Model file for the job. Use its own axes, mm. A direction names the side the tool comes from. Round coordinates to 2 decimals unless told otherwise and drop trailing zeros. Loops run counter-clockwise (first coordinate to the right, second up) from the corner with the lowest first, then second, coordinate; pieces in that order, holes last. Notation, with made-up numbers: M -10,53.5 L 48,53.5 A34 ccw 48,87.5 Z; hole C 67.5,-22.5 d1. An arc over 180 degrees is marked long. Answer in a Markdown table with one row per item.
from build123d import *

# Parameters (mm, degrees)
SKETCH1_W           = 229.616
SKETCH1_H           = 110.998
BOSS_EXTRUDE1_DEPTH = 12.7
DRAFT1_ANGLE        = -45
CUT_EXTRUDE1_DEPTH  = 139.893248743
CUT_EXTRUDE2_DEPTH  = 139.893248743


with BuildPart() as part:
    # Sketch1 → Boss-Extrude1 (new body)
    with BuildSketch(Plane(origin=(0, 0, 0), x_dir=(1, 0, 0), z_dir=(0, 1, 0))):
        with Locations((0, 21.631847801)):
            Rectangle(SKETCH1_W, SKETCH1_H)
    extrude(amount=BOSS_EXTRUDE1_DEPTH)

    # Draft1
    draft1_faces = [part.faces().sort_by_distance(p)[0] for p in [
        (-114.808, 6.35, -21.631847801),
        (114.808, 6.35, -21.631847801),
    ]]
    draft(draft1_faces, Plane.ZX.offset(12.7), DRAFT1_ANGLE)

    # Sketch2 → Cut-Extrude1 (cut, through all)
    with BuildSketch(Plane(origin=(0, 12.7, 0), x_dir=(1, 0, 0), z_dir=(0, 1, 0))):
        with BuildLine():
            Line((-114.808, -9.356152199), (-97.477466366, -9.356152199))
            ThreePointArc((-97.477466366, -9.356152199), (-88.138, -9.356152199), (-88.138, -18.695618565))
            Line((-88.138, -18.695618565), (-88.138, -33.867152199))
            Line((-88.138, -33.867152199), (-114.808, -33.867152199))
            Line((-114.808, -33.867152199), (-114.808, -9.356152199))
        make_face()
        with BuildLine():
            Line((114.808, -33.867152199), (114.808, -9.356152199))
            Line((114.808, -9.356152199), (97.477466366, -9.356152199))
            ThreePointArc((97.477466366, -9.356152199), (88.138, -9.356152199), (88.138, -18.695618565))
            Line((88.138, -18.695618565), (88.138, -33.867152199))
            Line((88.138, -33.867152199), (114.808, -33.867152199))
        make_face()
        with BuildLine():
            Line((84.224585113, 77.130847801), (114.808, 77.130847801))
            Line((114.808, 77.130847801), (114.808, 58.969847801))
            Line((114.808, 58.969847801), (91.336585113, 58.969847801))
            ThreePointArc((91.336585113, 58.969847801), (82.215723928, 60.978708985), (84.224585113, 70.099570169))
            Line((84.224585113, 70.099570169), (84.224585113, 77.130847801))
        make_face()
    extrude(amount=-CUT_EXTRUDE1_DEPTH, mode=Mode.SUBTRACT)

    # Sketch3 → Cut-Extrude2 (cut, through all)
    with BuildSketch(Plane(origin=(0, 12.7, 0), x_dir=(1, 0, 0), z_dir=(0, 1, 0))):
        with BuildLine():
            Line((-3.65376202, 52.971841669), (83.097055719, 45.380847801))
            ThreePointArc((83.097055719, 45.380847801), (88.989685458, 41.672106593), (89.408, 34.722080728))
            Line((89.408, 34.722080728), (67.818, -14.367006033))
            ThreePointArc((67.818, -14.367006033), (64.083911918, -18.195587555), (58.753320746, -18.627152199))
            Line((58.753320746, -18.627152199), (-6.407496993, -0.047071571))
            ThreePointArc((-6.407496993, -0.047071571), (-10.400202195, 2.69050833), (-11.938, 7.280847801))
            Line((-11.938, 7.280847801), (-11.938, 45.380847801))
            ThreePointArc((-11.938, 45.380847801), (-9.465956225, 50.99893882), (-3.65376202, 52.971841669))
        make_face()
    extrude(amount=-CUT_EXTRUDE2_DEPTH, mode=Mode.SUBTRACT)


solid = part.part
1. Saw through at A-A (y = 7.75). Write the cut outline in (x, z).
Verdict:
| item | result |
|---|---|
| outline | M -109.86,-77.13 L 84.22,-77.13 L 84.22,-70.1 A6.6 cw 91.34,-58.97 L 109.86,-58.97 L 109.86,9.36 L 97.48,9.36 A6.6 cw 88.14,18.7 L 88.14,33.87 L -88.14,33.87 L -88.14,18.7 A6.6 cw -97.48,9.36 L -109.86,9.36 Z; hole M -11.94,-45.38 A7.62 ccw -3.65,-52.97 L 83.1,-45.38 A7.62 ccw 89.41,-34.72 L 67.82,14.37 A7.62 ccw 58.75,18.63 L -6.41,0.05 A7.62 ccw -11.94,-7.28 Z |
2. Saw through at C-C (x = 44). Write the cut outline in (y, z).
Verdict:
| item | result |
|---|---|
| outline | M 0,-77.13 L 12.7,-77.13 L 12.7,-48.8 L 0,-48.8 Z; M 0,14.42 L 12.7,14.42 L 12.7,33.87 L 0,33.87 Z |
3. Wall check: probe 1 along X at (y, z) = (1.25, 24); probe 2 along Z at (x, y) = (-93, 7); probe 3 along X at (y, z) = (4.5, -38). Give the ranges that are in metal, low to high.
Verdict:
| item | result |
|---|---|
| probe 1 | x = -88.14 to 88.14 |
| probe 2 | z = -77.13 to 7.42 |
| probe 3 | x = -106.61 to -11.94, 90.05 to 106.61 |
4. Tool access for faces 1 (the flat face through (78.764, 6.439, -10.521)), 2 (the flat face through (-88.138, 6, 26)), 3 (the flat face through (84.225, 6, -74)): list every direction of +Z, -Z, +X, -X, +Y, -Y with a clear straight run to the whole face (end or side of a thin tool).
Verdict:
| item | result |
|---|---|
| face 1 | +Y, -Y |
| face 2 | +Z, -X, +Y, -Y |
| face 3 | -Z, +X, +Y, -Y |
5. Mould opens along Z. For faces 4 (the flat face through (-104, 8, 9.356)), 5 (the cylindrical face through (-88.242, 6.439, 9.255)), 6 (the cylindrical face through (88.242, 6.439, 9.255)), 7 (the flat face through (101, 8, -58.97)) say: +Z half, -Z half, draft (parallel to the pull), parting line (faces both ways), or undercut.
Verdict:
| item | result |
|---|---|
| face 4 | +Z half |
| face 5 | undercut |
| face 6 | undercut |
| face 7 | -Z half |
6. Saw through at D-D (z = 27.5). Write the cut outline in (x, y), and give its area (3 significant figures).
Verdict:
| item | result |
|---|---|
| outline | M -88.14,0 L 88.14,0 L 88.14,12.7 L -88.14,12.7 Z |
| area | 2,240 mm² |
7. Pin check, flat tips, straight feed: pin 1 (1 mm diameter, centred on y = 10, z = -65.5, fed in from +X); pin 2 (3 mm diameter, centred on y = 6.5, z = -48.5, fed in from +X); pin 3 (3.5 mm diameter, centred on y = 7, z = -72.5, fed in from +X). Stop position of each tip, or through.
Verdict:
| item | result |
|---|---|
| pin 1 | stops at x = 81.34 |
| pin 2 | stops at x = 110.11 |
| pin 3 | stops at x = 84.22 |
8. Saw through at B-B (z = 3). Write the cut outline in (x, y), and give its area (3 significant figures).
Verdict:
| item | result |
|---|---|
| outline | M -114.81,12.7 L -102.11,0 L 3.95,0 L 3.95,12.7 Z; M 72.82,0 L 102.11,0 L 114.81,12.7 L 72.82,12.7 Z |
| area | 1,880 mm² |
